Design review of the part built by this model. Coordinates are the model's own, in mm. A direction names the side the tool comes from. Coordinates: 2 decimals unless noted, no trailing zeros. Write each loop counter-clockwise with the first axis right and the second up, starting at its lowest first coordinate (ties: lowest second). Pieces come first, ordered by that corner, then holes.
Q1. To check wall thickness, follow probe 1 along X at (y, z) = (1.95, -40.5); probe 2 along X at (y, z) = (0.95, -44); probe 3 along Z at (x, y) = (-31, 2). State the ranges of each line that lie inside material, in increasing order.
Q2. Add section B-B, the plane x = -31.5. Give the boundary of the cut face in (y, z), plus the area to 3 significant figures.
Q3. Add section A-A, the plane z = -44. Give the boundary of the cut face in (x, y).
Q4. Add section C-C, the plane y = -40. Give the boundary of the cut face in (x, z), plus the area to 3 significant figures.
Q5. Machinability: for faces 5 (the face through (-38, 1, -35.5)), 6 (the face through (21.794, -30, -7)), 7 (the face through (30, -60, -29)), 8 (the face through (27, -32, 5.337)), which of the approach directions +Z, -Z, +X, -X, +Y, -Y give a long, thin tool a straight path to every point of the face, cutting with its end or side? Answer none if there is none.
Q6. Clearance check with flat-ended pins moving along their axes: pin 1 Ø3 at (y, z) = (-30, 25.5) entering from -X; pin 2 Ø8 at (x, y) = (24.5, -42) entering from +Z; pin 3 Ø1.9 at (x, y) = (27.5, -67) entering from -Z. State where each tip first meets the part, or that it passes through.
Q7. The part is to be moulded in two halves that separate along Z. For faces 1 (the face through (-1, 1, 50)), 2 (the face through (50, 1, 1)), 3 (the face through (27, -32, -30.5)), 4 (the face through (27, -32, -20.5)), say which applies: +Z half, -Z half, draft (parallel to the pull), parting line (faces both ways), or undercut.
Q8. Add section D-D, the plane x = 44. Give the boundary of the cut face in (y, z), plus the area to 3 significant figures.
from build123d import *

# Parameters (mm, degrees)
CROQUIS1_W              = 100
CROQUIS1_H              = 100
SALIENTE_EXTRUIR1_DEPTH = 3
CROQUIS6_R              = 1.55
CORTAR_EXTRUIR4_DEPTH   = 10
CROQUIS7_R              = 1.6
CORTAR_EXTRUIR5_DEPTH   = 10
CROQUIS8_W              = 3
CROQUIS8_H              = 100
SALIENTE_EXTRUIR3_DEPTH = 3
CROQUIS9_W              = 10
CROQUIS9_H              = 61
SALIENTE_EXTRUIR4_DEPTH = 60
CROQUIS10_W             = 4.321859215
CROQUIS10_H             = 55
SALIENTE_EXTRUIR5_DEPTH = 10
CROQUIS11_W             = 55
CROQUIS11_H             = 3
SALIENTE_EXTRUIR6_DEPTH = 2
SALIENTE_EXTRUIR7_DEPTH = 61
CROQUIS13_W             = 10
CROQUIS13_H             = 71
CORTAR_EXTRUIR6_DEPTH   = 61
CROQUIS14_W             = 10
CROQUIS14_H             = 49
CORTAR_EXTRUIR7_DEPTH   = 61


with BuildPart() as part:
    # Croquis1 → Saliente-Extruir1 (new body)
    with BuildSketch(Plane(origin=(0, 0, 0), x_dir=(1, 0, 0), z_dir=(0, 1, 0))):
        Rectangle(CROQUIS1_W, CROQUIS1_H)
    extrude(amount=SALIENTE_EXTRUIR1_DEPTH)

    # Croquis6 → Cortar-Extruir4 (cut)
    with BuildSketch(Plane(origin=(0, 3, 0), x_dir=(1, 0, 0), z_dir=(0, 1, 0))):
        with Locations(Location((-44, 44, 0), (0, 0, 270))):  # turned: the seam where the file's is
            Circle(CROQUIS6_R)
        with Locations(Location((44, 44, 0), (0, 0, 270))):  # turned: the seam where the file's is
            Circle(CROQUIS6_R)
        with Locations(Location((44, -44, 0), (0, 0, 270))):  # turned: the seam where the file's is
            Circle(CROQUIS6_R)
        with Locations(Location((-44, -44, 0), (0, 0, 270))):  # turned: the seam where the file's is
            Circle(CROQUIS6_R)
    extrude(amount=-CORTAR_EXTRUIR4_DEPTH, mode=Mode.SUBTRACT)

    # Croquis7 → Cortar-Extruir5 (cut)
    with BuildSketch(Plane(origin=(0, 3, 0), x_dir=(1, 0, 0), z_dir=(0, 1, 0))):
        with Locations(Location((-31.5, 40.5, 0), (0, 0, 270))):  # turned: the seam where the file's is
            Circle(CROQUIS7_R)
        with Locations(Location((31.5, 40.5, 0), (0, 0, 270))):  # turned: the seam where the file's is
            Circle(CROQUIS7_R)
        with Locations(Location((-31.5, -40.5, 0), (0, 0, 270))):  # turned: the seam where the file's is
            Circle(CROQUIS7_R)
        with Locations(Location((31.5, -40.5, 0), (0, 0, 270))):  # turned: the seam where the file's is
            Circle(CROQUIS7_R)
    extrude(amount=-CORTAR_EXTRUIR5_DEPTH, mode=Mode.SUBTRACT)

    # Croquis8 → Saliente-Extruir3 (add)
    with BuildSketch(Plane.XZ):
        with Locations((-48.5, 0)):
            Rectangle(CROQUIS8_W, CROQUIS8_H)
    extrude(amount=SALIENTE_EXTRUIR3_DEPTH)

    # Croquis9 → Saliente-Extruir4 (add)
    with BuildSketch(Plane.XZ):
        with Locations((26.793549779, 0)):
            Rectangle(CROQUIS9_W, CROQUIS9_H)
    extrude(amount=SALIENTE_EXTRUIR4_DEPTH)

    # Croquis10 → Saliente-Extruir5 (add)
    with BuildSketch(Plane.XZ.offset(60)):
        with Locations((29.632620172, 0)):
            Rectangle(CROQUIS10_W, CROQUIS10_H)
    extrude(amount=SALIENTE_EXTRUIR5_DEPTH)

    # Croquis11 → Saliente-Extruir6 (add)
    with BuildSketch(Plane.ZY.offset(-27.471690564)):
        with Locations((0, -68.5)):
            Rectangle(CROQUIS11_W, CROQUIS11_H)
    extrude(amount=SALIENTE_EXTRUIR6_DEPTH)

    # Croquis12 → Saliente-Extruir7 (add)
    with BuildSketch(Plane.XY.offset(30.5)):
        Polygon((21.793549779, -60), (27.471690564, -60), (27.471690564, -65.263594713), align=None)
        Polygon((-44.699438936, -1.906763457), (-47, -1.906763457), (-47, 0), (-42.931883245, 0), align=None)
    extrude(amount=-SALIENTE_EXTRUIR7_DEPTH)

    # Croquis13 → Cortar-Extruir6 (cut)
    with BuildSketch(Plane.XZ):
        with Locations((-37.931883245, 0)):
            Rectangle(CROQUIS13_W, CROQUIS13_H)
    extrude(amount=-CORTAR_EXTRUIR6_DEPTH, mode=Mode.SUBTRACT)

    # Croquis14 → Cortar-Extruir7 (cut)
    with BuildSketch(Plane(origin=(31.793549779, 0, 0), x_dir=(0, 0, -1), z_dir=(1, 0, 0))):
        with Locations((-15.5, -31.474245952)):
            Rectangle(CROQUIS14_W, CROQUIS14_H)
        with Locations((-0.336542235, -31.474245952)):
            Rectangle(CROQUIS14_W, CROQUIS14_H)
        with Locations((15.5, -31.474245952)):
            Rectangle(CROQUIS14_W, CROQUIS14_H)
    extrude(amount=-CORTAR_EXTRUIR7_DEPTH, mode=Mode.SUBTRACT)


solid = part.part
Here are the results:
1. probe 1: x = -50 to -33.1, -29.9 to 29.9, 33.1 to 50
1. probe 2: x = -50 to -45.55, -42.45 to 42.45, 45.55 to 50
1. probe 3: z = -50 to -42.02, -38.98 to 38.98, 42.02 to 50
2. outline: (0, -50) - (3, -50) - (3, -42.1) - (0, -42.1) - close; (0, -38.9) - (3, -38.9) - (3, 38.9) - (0, 38.9) - close; (0, 42.1) - (3, 42.1) - (3, 50) - (0, 50) - close
2. area: 281 mm2
3. outline: (-50, -3) - (-47, -3) - (-47, 0) - (-45.55, 0) - (-45.55, 3) - (-50, 3) - close; (-42.45, 0) - (42.45, 0) - (42.45, 3) - (-42.45, 3) - close; (45.55, 0) - (50, 0) - (50, 3) - (45.55, 3) - close
4. outline: (21.79, -30.5) - (31.79, -30.5) - (31.79, -20.5) - (21.79, -20.5) - close; (21.79, -10.5) - (31.79, -10.5) - (31.79, -4.66) - (21.79, -4.66) - close; (21.79, 5.34) - (31.79, 5.34) - (31.79, 10.5) - (21.79, 10.5) - close; (21.79, 20.5) - (31.79, 20.5) - (31.79, 30.5) - (21.79, 30.5) - close
4. area: 310 mm2
5. face 5: +Y, -Y
5. face 6: +Z, -Z, -Y
5. face 7: -Z, +X, -Y
5. face 8: +X, -X
6. pin 1: stops at x = 21.79
6. pin 2: stops at z = 30.5
6. pin 3: stops at z = -27.5
7. face 1: +Z half
7. face 2: draft
7. face 3: -Z half
7. face 4: undercut
8. outline: (0, -50) - (3, -50) - (3, -45.55) - (0, -45.55) - close; (0, -42.45) - (3, -42.45) - (3, 42.45) - (0, 42.45) - close; (0, 45.55) - (3, 45.55) - (3, 50) - (0, 50) - close
8. area: 281 mm2
